Geometry: final body of the model. Coordinates: model frame, mm. A direction names the side the tool comes from. Coordinates: 2 decimals unless noted, no trailing zeros. Order: outer loops, then holes, each group sorted by start corner. A loop starts at its lowest first (then second) coordinate and runs counter-clockwise, first axis right, second up. Notation, with made-up numbers: M 4,-22.75 L 38,-22.75 A22 cw 38,7.25 Z; hole C 39.5,42 d10. An arc over 180 degrees is marked long. Use CSV: the item, a comma, the result in double quotes. Start each with the question number.
Q1. Section query C-C, the plane z = 16. Output: boundary loops of the cut face in (x, y).
Q2. Access query for faces 1 (the face through (-6.094, 0.268, 4.93)), 2 (the face through (-0.867, -3.905, 14.951)), 3 (the face through (0, 0, 0)). Directions: +Z, -Z, +X, -X, +Y, -Y. A direction counts if a zero-diameter tool reaches every point of the face in a straight line with its end or side. Return the directions, or none.
Q3. Ray query, probe 1 along Z at (x, y) = (1, 5.5); probe 2 along Z at (x, y) = (7, 0.75); probe 3 along Y at (x, z) = (-0.25, 3.75). Return the intervals inside material, ascending.
Q4. Section query A-A, the plane y = 0. Output: boundary loops of the cut face in (x, z).
Q5. First-contact query: P1, Ø2, axis at x = -3.5, y = 0.5, coming from the -Z side; P2, Ø3, axis at x = 4, z = 2, coming from the +Y side; P3, Ø4, axis at y = 5, z = 15, coming from the -X side; P4, Ø1.5, axis at x = 5, z = 6.5, coming from the +Y side. Flat tips, straight axial feed; report the tip coordinate or a pass-through.
Q6. Section query D-D, the plane x = 5.75. Output: boundary loops of the cut face in (y, z), and give its area (3 significant figures).
from build123d import *

# Parameters (mm, degrees)
F0_R     = 6.1
F0_R_2   = 4
F1_DEPTH = 10
F2_DEPTH = 18.5
F3_R     = 8
F4_DEPTH = 1.5


with BuildPart() as f1:
    # F0 (on Top) → F1 (new body)
    with BuildSketch(Plane.XY):
        Circle(F0_R)
        Circle(F0_R_2, mode=Mode.SUBTRACT)
    extrude(amount=F1_DEPTH)

    # F0 (on Top) → F2 (join)
    with BuildSketch(Plane.XY):
        Circle(F0_R_2)
    extrude(amount=F2_DEPTH)

    # F3 (on face) → F4 (join)
    with BuildSketch(Plane.XY.offset(10)):
        Circle(F3_R)
    extrude(amount=F4_DEPTH)


solid = f1.part
Responses:
1,outline,"C 0,0 d8"
2,face 1,"-Z"
2,face 2,"+Z"
2,face 3,"-Z, +X, -X, +Y, -Y"
3,probe 1,"z = 0 to 11.5"
3,probe 2,"z = 10 to 11.5"
3,probe 3,"y = -6.09 to 6.09"
4,outline,"M -8,10 L -6.1,10 L -6.1,0 L 6.1,0 L 6.1,10 L 8,10 L 8,11.5 L 4,11.5 L 4,18.5 L -4,18.5 L -4,11.5 L -8,11.5 Z"
5,P1,"stops at z = 0"
5,P2,"stops at y = 5.56"
5,P3,"stops at x = -2.65"
5,P4,"stops at y = 4.38"
6,outline,"M -5.56,10 L -2.04,10 L -2.04,0 L 2.04,0 L 2.04,10 L 5.56,10 L 5.56,11.5 L -5.56,11.5 Z"
6,area,"57.4 mm²"
